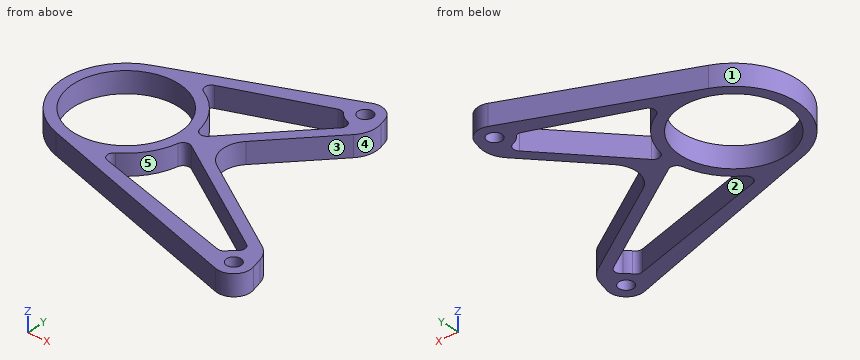
```python
from build123d import *

# Parameters (mm, degrees)
SKETCH4_R           = 40
SKETCH4_R_2         = 5.5
BOSS_EXTRUDE1_DEPTH = 15.875
CUT_EXTRUDE2_DEPTH  = 265.729718277
FILLET1_R           = 5
CUT_EXTRUDE3_DEPTH  = 265.729718424
FILLET2_R           = 20


with BuildPart() as part:
    # Sketch4 → Boss-Extrude1 (new body)
    with BuildSketch(Plane.XY):
        with BuildLine():
            Line((-142.633865887, -146.080164327), (21.544941406, -195.965223983))
            ThreePointArc((21.544941406, -195.965223983), (33.862932788, -192.99616638), (37.258075063, -180.78874144))
            Line((37.258075063, -180.78874144), (-7.649527095, -12.138772571))
            ThreePointArc((-7.649527095, -12.138772571), (-14.239674224, -4.124786339), (-24.611636772, -3.848367419))
            Line((-24.611636772, -3.848367419), (-147.429933804, -55.967315581))
            ThreePointArc((-147.429933804, -55.967315581), (-176.611366682, -102.704491033), (-142.633865887, -146.080164327))
        make_face()
        with Locations((-128.679206861, -100.153402069)):
            Circle(SKETCH4_R, mode=Mode.SUBTRACT)
        with Locations((25.178967194, -184.005129645)):
            Circle(SKETCH4_R_2, mode=Mode.SUBTRACT)
        with Locations((-19.728634964, -15.355160776)):
            Circle(SKETCH4_R_2, mode=Mode.SUBTRACT)
    extrude(amount=BOSS_EXTRUDE1_DEPTH)

    # Sketch5 → Cut-Extrude2 (cut, through all)
    with BuildSketch(Plane.XY.offset(15.875)):
        with BuildLine():
            Line((-31.394262991, -19.845497372), (-118.286356862, -53.292024914))
            ThreePointArc((-118.286356862, -53.292024914), (-91.243550062, -70.110572642), (-80.679206861, -100.153402069))
            Line((-80.679206861, -100.153402069), (-10.524781522, -23.813238679))
            ThreePointArc((-10.524781522, -23.813238679), (-22.063335437, -27.635192278), (-31.394262991, -19.845497372))
        make_face()
        with BuildLine():
            ThreePointArc((-80.708447165, -101.828577911), (-90.303653302, -128.985968536), (-113.716587883, -145.761735006))
            Line((-113.716587883, -145.761735006), (13.127445592, -180.686873014))
            ThreePointArc((13.127445592, -180.686873014), (20.684837316, -172.340962438), (31.888396226, -173.458397351))
            Line((31.888396226, -173.458397351), (-80.708447165, -101.828577911))
        make_face()
    extrude(amount=-CUT_EXTRUDE2_DEPTH, mode=Mode.SUBTRACT)

    # Fillet1
    fillet1_edges = [part.edges().sort_by_distance(p)[0] for p in [
        (-31.394262991, -19.845497372, 7.9375),
        (-10.524781522, -23.813238679, 7.9375),
        (-80.679206861, -100.153402069, 7.9375),
        (-118.286356862, -53.292024914, 7.9375),
        (13.127445592, -180.686873014, 7.9375),
        (-113.716587883, -145.761735006, 7.9375),
        (-80.708447165, -101.828577911, 7.9375),
    ]]
    fillet(fillet1_edges, radius=FILLET1_R)
    fillet1_2_edges = [part.edges().sort_by_distance(p)[0] for p in [
        (31.888396226, -173.458397351, 7.9375),
    ]]
    fillet(fillet1_2_edges, radius=FILLET1_R)

    # Sketch6 → Cut-Extrude3 (cut, through all)
    with BuildSketch(Plane.XY.offset(15.875)):
        Polygon((-69.306214403, -99.600633953), (-3.444297399, -27.931462965), (32.963567977, -164.660770859), align=None)
    extrude(amount=-CUT_EXTRUDE3_DEPTH, mode=Mode.SUBTRACT)

    # Fillet2
    fillet2_edges = [part.edges().sort_by_distance(p)[0] for p in [
        (32.963567977, -164.660770859, 7.9375),
        (-69.306214403, -99.600633953, 7.9375),
        (-3.444297399, -27.931462965, 7.9375),
    ]]
    fillet(fillet2_edges, radius=FILLET2_R)


solid = part.part
```
The listing builds one solid part. Answer for the finished solid, in the listing's coordinates (mm). Face numbers are marked on the shaded views. A direction names the side the tool comes from. Give positions to 0.01 mm unless a question says otherwise; leave off trailing zeros. Order: outer loops, then holes, each group sorted by start corner. A loop starts at its lowest first (then second) coordinate and runs counter-clockwise, first axis right, second up. Notation, with made-up numbers: (-10.75, -21) -> (20.25, -21) arc R10 ccw to (20.25, -8) -> close; hole circle Ø11 at (21, 65.25). An arc over 180 degrees is marked (long way). One line per item, written item: value.
1) Find section A-A, the plane y = -135. Determine the outline of the cut face in (x, z) (3 decimals).
Reported:
outline: (-161.69, 0) -> (-148.319, 0) -> (-148.319, 15.875) -> (-161.69, 15.875) -> close; (-109.04, 0) -> (-95.668, 0) -> (-95.668, 15.875) -> (-109.04, 15.875) -> close; (-28.565, 0) -> (-13.661, 0) -> (-13.661, 15.875) -> (-28.565, 15.875) -> close
2) Flat-ended cylindrical pins translate along their axes: P1, Ø5, axis at y = -113, z = 6.5, coming from the +X side; P2, Ø1.5, axis at y = -47, z = 1.5, coming from the +X side; P3, Ø1.5, axis at y = -92, z = 7, coming from the -X side. Find the tip coordinate at first contact, or state that the pin passes through.
Reported:
P1: stops at x = -44.31
P2: stops at x = -20.28
P3: stops at x = -176.1
3) Find section C-C, the plane z = 11.75. Count the separate pieces of the cut face and the enclosed holes in it, plus the area to 3 significant figures.
Reported:
separate pieces: 1
enclosed holes: 5
area: 7,730 mm^2
4) Find section D-D, the plane y = -167.5. Determine the outline of the cut face in (x, z) (3 decimals), plus the area to 3 significant figures.
Reported:
outline: (-72.138, 0) -> (-34.766, 0) -> (-34.766, 15.875) -> (-72.138, 15.875) -> close; (20.57, 0) -> (33.053, 0) -> (33.053, 15.875) -> (20.57, 15.875) -> close
area: 791 mm^2
5) Find section B-B, the plane x = -119.5. Determine the outline of the cut face in (y, z) (3 decimals).
Reported:
outline: (-153.109, 0) -> (-139.086, 0) -> (-139.086, 15.875) -> (-153.109, 15.875) -> close; (-61.221, 0) -> (-44.115, 0) -> (-44.115, 15.875) -> (-61.221, 15.875) -> close
6) Find the intervals of material crossed by line 1 (Y direction, x = -38, z = 1.75); line 2 (X direction, y = -73.5, z = 11.75); line 3 (X direction, y = -69, z = 6.5), in increasing order.
Reported:
line 1: y = -177.87 to -166.61, -129 to -119.52, -65.53 to -53.71, -22.39 to -9.53
line 2: x = -168.6 to -158.51, -98.85 to -88.76, -56.19 to -45.32
line 3: x = -165.2 to -153.77, -103.59 to -92.16, -52.05 to -41.19
7) A tool of negligible diameter and unlimited length cuts with its end or side. For the marked faces 4 and 5, from which of +Z, -Z, +X, -X, +Y, -Y can it reach the whole face along a straight path? Write none if from no direction.
Reported:
face 4: +Z, -Z, +X
face 5: +Z, -Z
8) Determine the mould class of the marked faces 1, 2 and 3 for opening direction X: pulls with the +X half, pulls with the -X half, needs draft (parallel to the pull), parting line crosses it, or undercut.
Reported:
face 1: pulls with the -X half
face 2: undercut
face 3: pulls with the +X half
